Check sheet for the modelled part. Datum: model origin and axes. Units: mm. A direction names the side the tool comes from. Give positions to 0.01 mm unless a question says otherwise; leave off trailing zeros. Loops run counter-clockwise (first coordinate to the right, second up) from the corner with the lowest first, then second, coordinate; pieces in that order, holes last. Notation, with made-up numbers: (1.25, 73.25) - (18.25, 73.25) arc R28 cw to (18.25, 106.25) - close; hole circle Ø7 at (-33, 72). An arc over 180 degrees is marked (long way). Use one line per item in the form item = value.
from build123d import *

# Parameters (mm, degrees)
SKETCH1_W           = 25
SKETCH1_H           = 12.5
BOSS_EXTRUDE1_DEPTH = 5
FILLET1_R           = 2
SKETCH4_R           = 1.5
CUT_EXTRUDE1_DEPTH  = 21.310096012
SKETCH5_W           = 17
SKETCH5_H           = 8.5
CUT_EXTRUDE2_DEPTH  = 2.5
BOSS_EXTRUDE2_DEPTH = 5


with BuildPart() as part:
    # Sketch1 → Boss-Extrude1 (new body)
    with BuildSketch(Plane(origin=(0, 0, 0), x_dir=(1, 0, 0), z_dir=(0, 1, 0))):
        Rectangle(SKETCH1_W, SKETCH1_H)
    extrude(amount=BOSS_EXTRUDE1_DEPTH)

    # Sketch3 → Revolve1 (revolve)
    with BuildSketch(Plane.XY):
        Polygon((-6.75, 5), (-7.5, 5), (-7.5, 6), (-8.25, 6), (-8.25, 7), (-7.495786155, 7), (-7.495786155, 8.5), (-8.25, 8.5), (-6.75, 10), align=None)
    revolve1 = revolve(axis=Axis((-6.25, 11.553372133, 0), (0, -1, 0)))

    # Fillet1
    fillet1_edges = [part.edges().sort_by_distance(p)[0] for p in [
        (12.5, 5, 0),
        (-12.5, 5, 0),
        (12.5, 0, 0),
        (-12.5, 0, 0),
    ]]
    fillet(fillet1_edges, radius=FILLET1_R)

    # Sketch4 → Cut-Extrude1 (cut, through all)
    with BuildSketch(Plane(origin=(0, 0, -6.25), x_dir=(-1, 0, 0), z_dir=(0, 0, -1))):
        with Locations((10.5, 2.5)):
            Circle(SKETCH4_R)
        with Locations((-10.5, 2.5)):
            Circle(SKETCH4_R)
    extrude(amount=-CUT_EXTRUDE1_DEPTH, mode=Mode.SUBTRACT)

    # Mirror1: Revolve1 across plane
    add(revolve1.mirror(Plane(origin=(0, 0, 0), x_dir=(0, 0, 1), z_dir=(1, 0, 0))))

    # Sketch5 → Cut-Extrude2 (cut)
    with BuildSketch(Plane.XZ):
        Rectangle(SKETCH5_W, SKETCH5_H)
    extrude(amount=-CUT_EXTRUDE2_DEPTH, mode=Mode.SUBTRACT)

    # Sketch6 → Boss-Extrude2 (add)
    with BuildSketch(Plane.XZ.offset(-2.5)):
        with BuildLine():
            Line((0.5, 0.15), (0.5, 0.85))
            ThreePointArc((0.5, 0.85), (0.543933983, 0.956066017), (0.65, 1))
            Line((0.65, 1), (1.35, 1))
            ThreePointArc((1.35, 1), (1.456066017, 0.956066017), (1.5, 0.85))
            Line((1.5, 0.85), (1.5, 0.15))
            ThreePointArc((1.5, 0.15), (1.456066017, 0.043933983), (1.35, 0))
            Line((1.35, 0), (0.65, 0))
            ThreePointArc((0.65, 0), (0.543933983, 0.043933983), (0.5, 0.15))
        make_face()
        with BuildLine():
            Line((2.65, 0), (3.35, 0))
            ThreePointArc((3.35, 0), (3.456066017, 0.043933983), (3.5, 0.15))
            Line((3.5, 0.15), (3.5, 0.85))
            ThreePointArc((3.5, 0.85), (3.456066017, 0.956066017), (3.35, 1))
            Line((3.35, 1), (2.65, 1))
            ThreePointArc((2.65, 1), (2.543933983, 0.956066017), (2.5, 0.85))
            Line((2.5, 0.85), (2.5, 0.15))
            ThreePointArc((2.5, 0.15), (2.543933983, 0.043933983), (2.65, 0))
        make_face()
        with BuildLine():
            Line((-1.5, 0.15), (-1.5, 0.85))
            ThreePointArc((-1.5, 0.85), (-1.456066017, 0.956066017), (-1.35, 1))
            Line((-1.35, 1), (-0.65, 1))
            ThreePointArc((-0.65, 1), (-0.543933983, 0.956066017), (-0.5, 0.85))
            Line((-0.5, 0.85), (-0.5, 0.15))
            ThreePointArc((-0.5, 0.15), (-0.543933983, 0.043933983), (-0.65, 0))
            Line((-0.65, 0), (-1.35, 0))
            ThreePointArc((-1.35, 0), (-1.456066017, 0.043933983), (-1.5, 0.15))
        make_face()
        with BuildLine():
            Line((-3.5, 0.15), (-3.5, 0.85))
            ThreePointArc((-3.5, 0.85), (-3.456066017, 0.956066017), (-3.35, 1))
            Line((-3.35, 1), (-2.65, 1))
            ThreePointArc((-2.65, 1), (-2.543933983, 0.956066017), (-2.5, 0.85))
            Line((-2.5, 0.85), (-2.5, 0.15))
            ThreePointArc((-2.5, 0.15), (-2.543933983, 0.043933983), (-2.65, 0))
            Line((-2.65, 0), (-3.35, 0))
            ThreePointArc((-3.35, 0), (-3.456066017, 0.043933983), (-3.5, 0.15))
        make_face()
    extrude(amount=BOSS_EXTRUDE2_DEPTH)


solid = part.part
Item 1: Section check C-C on y = 9.25. Record the boundary of the cut face in (x, z).
Answer block:
outline = circle Ø2.5 at (-6.25, 0); circle Ø2.5 at (6.25, 0); hole circle Ø1 at (-6.25, 0); hole circle Ø1 at (6.25, 0)
Item 2: Section check A-A on z = -4.75. Record the boundary of the cut face in (x, y).
Answer block:
outline = (-12.5, 2) arc R2 ccw to (-10.5, 0) - (10.5, 0) arc R2 ccw to (12.5, 2) - (12.5, 3) arc R2 ccw to (10.5, 5) - (-10.5, 5) arc R2 ccw to (-12.5, 3) - close; hole circle Ø3 at (-10.5, 2.5); hole circle Ø3 at (10.5, 2.5)
Item 3: Gauge pin test, flat ends, axial feed: P1, Ø0.6, axis at y = -1, z = 0.5, coming from the +X side; P2, Ø0.6, axis at y = 0.5, z = 0.5, coming from the +X side; P3, Ø2, axis at x = -8.5, z = -1.5, coming from the +Y side. Record the tip position at first contact, or that the pin passes through.
Answer block:
P1 = 3.5
P2 = 12.1
P3 = 8.8
Item 4: Thickness scan on L1, parallel to X at y = 7.45, z = 0; L2, parallel to X at y = -2, z = 0.75; L3, parallel to Z at x = -6.25, y = 8.3. Record the ranges inside material, lowest first.
Answer block:
L1 = -7.5 to -6.75, -5.75 to -5, 5 to 5.75, 6.75 to 7.5
L2 = -3.5 to -2.5, -1.5 to -0.5, 0.5 to 1.5, 2.5 to 3.5
L3 = -1.25 to -0.5, 0.5 to 1.25
Item 5: Section check D-D on x = -6.25. Record the boundary of the cut face in (y, z), then the cut area to 3 significant figures.
Answer block:
outline = (0, -6.25) - (5, -6.25) - (5, -1.25) - (6, -1.25) - (6, -2) - (7, -2) - (7, -1.25) - (8.5, -1.25) - (8.5, -2) - (10, -0.5) - (5, -0.5) - (5, 0.5) - (10, 0.5) - (8.5, 2) - (8.5, 1.25) - (7, 1.25) - (7, 2) - (6, 2) - (6, 1.25) - (5, 1.25) - (5, 6.25) - (0, 6.25) - (0, 4.25) - (2.5, 4.25) - (2.5, -4.25) - (0, -4.25) - close
area = 50.2 mm2
Item 6: Access from +Z, -Z, +X, -X, +Y, -Y to the whole of each face (thin tool, end or side, straight path). Record for faces 1 (the face through (-6, 5, 0)), 2 (the face through (0, 2.5, 0)), 3 (the face through (-11.93, 0.6, -0.09)), 4 (the face through (-5, 6, -1)).
Answer block:
face_1 = +Y
face_2 = -Y
face_3 = +Z, -Z, -X, -Y
face_4 = none
Item 7: Section check B-B on y = -0.75. Give the number of separate pieces and of enclosed holes in the cut face, then the cut area to 3 significant figures.
Answer block:
separate_pieces = 4
enclosed_holes = 0
area = 3.92 mm2
Item 8: Mould release check, pull along Z, two halves, no side actions. Record for faces 5 (the face through (12.5, 2.5, 0.1)), 6 (the face through (0, 2, -6.25)), 7 (the face through (-5.75, 7.46, -0.02)): released by +Z, released by -Z, zero draft, split by the parting line, or undercut.
Answer block:
face_5 = zero draft
face_6 = released by -Z
face_7 = undercut
